Source: CAD feature listing. Evaluate the final solid. Frame: model axes, mm. Give positions to 0.01 mm unless a question says otherwise; leave off trailing zeros. Write each loop counter-clockwise with the first axis right and the second up, starting at its lowest first coordinate (ties: lowest second). Pieces come first, ordered by that corner, then holes.
```python
from build123d import *

# Parameters (mm, degrees)
F0_R          = 31.2169949435
F1_DEPTH      = 25
F3_DEPTH      = 44
F3_TAPER      = -3
F3_DEPTH_BACK = 25


with BuildPart() as f1:
    # F0 (on Front) → F1 (new body)
    with BuildSketch(Plane.XZ):
        with Locations((23.8612815738, -5.9305061586)):
            Circle(F0_R)
    extrude(amount=F1_DEPTH)


with BuildPart() as f3:
    # F2 (on Top) → F3 (new body, two sides)
    with BuildSketch(Plane.XY) as f3_sk:
        Polygon((21.6927394478, -5.0327842001), (16.6236866582, 13.8126411778), (-2.2314568589, 18.8454253778), (-16.0175475864, 5.0327842001), (-10.9484947969, -13.8126411778), (7.9066487202, -18.8454253778), align=None)
    extrude(amount=F3_DEPTH, taper=F3_TAPER)
    extrude(f3_sk.sketch, amount=-F3_DEPTH_BACK)


with BuildPart() as f1_1:
    add(f1.part)

    # F4: cut F3
    add(f3.part, mode=Mode.SUBTRACT)


solid = f1_1.part
```
1. Section query B-B (x = 32.5). Return loops of the section in (y, z), plus the area to 3 significant figures.
2. Section query D-D (z = -27). Return loops of the section in (x, y).
3. Pull-direction query (Y, two-part tool) for faces 1 (the flat face through (21.025, -2.552, -12.325)), 2 (the flat face through (0.17, -16.78, -12.32)), 3 (the flat face through (23, -25, -5)); classes: pulls with the +Y half, pulls with the -Y half, needs draft (parallel to the pull), parting line crosses it, or undercut.
4. Pin query (flat end, axial travel): P1, Ø6, axis at y = -16, z = 0.5, coming from the -X side; P2, Ø3, axis at x = 41, y = -12.5, coming from the +Z side; P3, Ø2, axis at y = -18.5, z = -18.5, coming from the -X side. Return the tip coordinate at first contact, or that it passes through.
5. Section query C-C (y = -21.25). Return loops of the section in (x, z), plus the area to 3 significant figures.
6. Line query: probe 1 along Z at (x, y) = (2.5, -15); probe 2 along Z at (x, y) = (16, -6.5); probe 3 along Y at (x, z) = (20, -16.5). Output: solid intervals per line, ascending.
7. Section query A-A (z = -20.5). Return loops of the section in (x, y), plus the area to 3 significant figures.
The answers:
1. outline: (-25, -35.93) - (0, -35.93) - (0, 24.07) - (-25, 24.07) - close
1. area: 1,500 mm2
2. outline: (0.83, -25) - (46.9, -25) - (46.9, 0) - (0.83, 0) - close
3. face 1: undercut
3. face 2: pulls with the +Y half
3. face 3: pulls with the -Y half
4. P1: stops at x = -7.17
4. P2: stops at z = 21.09
4. P3: stops at x = -5.13
5. outline: circle Ø62.43 at (23.86, -5.93)
5. area: 3,060 mm2
6. probe 1: z = -28.69 to -25
6. probe 2: z = -36.14 to -25
6. probe 3: y = -25 to -6.73
7. outline: (-3.75, -25) - (51.47, -25) - (51.47, 0) - (20.34, 0) - (21.69, -5.03) - (7.91, -18.85) - (-3.75, -15.73) - close
7. area: 1,020 mm2
